Design review of the part built by this model. Coordinates are the model's own, in mm. A direction names the side the tool comes from. Coordinates: 2 decimals unless noted, no trailing zeros. Write each loop counter-clockwise with the first axis right and the second up, starting at its lowest first coordinate (ties: lowest second). Pieces come first, ordered by that corner, then holes.
Q1. Take a section at B-B, the plane x = -99. Write out the cut boundary in (y, z), plus the area to 3 significant figures.
Q2. For faces 1 (the flat face through (-185, -4, 5.452)), 2 (the flat face through (192.4, 0.1, -17.3)), 3 (the flat face through (177.6, 0.1, -0.1)), list the 3-axis set-ups (+Z, -Z, +X, -X, +Y, -Y) from which the entire face can be reached by the end or side of a thin tool; tool diameter is ignored.
Q3. The part is to be moulded in two halves that separate along Z. For faces 4 (the flat face through (-3, -3, -30)), 5 (the flat face through (187, -2, 5)), 6 (the flat face through (-3, 0, 30)), 7 (the flat face through (-3, 7.5, 3)), say which applies: released by +Z, released by -Z, zero draft, split by the parting line, or undercut.
Q4. For L1, parallel to Z at x = 182, y = -1.25; L2, parallel to Z at x = 152.5, y = 4; L3, parallel to Y at x = -55.5, z = -26.5, list the stretches that pass through material, from the lowest coordinate up.
Q5. For pin 1 Ø1 at (y, z) = (-4, -20) entering from +X; pin 2 Ø3 at (y, z) = (0.5, 20.5) entering from +X; pin 3 Ø1 at (y, z) = (0.5, 17.5) entering from -X, all flat-tipped, find the tip position at first contact; note any pin that passes through.
Q6. Take a section at A-A, the plane y = -0.25. Write out the cut boundary in (x, z), plus the area to 3 significant figures.
Q7. Take a section at C-C, the plane z = 13.5. Write out the cut boundary in (x, y), plus the area to 4 significant figures.
from build123d import *

# Parameters (mm, degrees)
F0_W     = 400
F0_H     = 60
F1_DEPTH = 7.5
F3_DEPTH = 60
F4_W     = 21.213203
F4_H     = 10
F5_DEPTH = 25
F6_W     = 21.213203
F6_H     = 10.904174
F7_DEPTH = 25
F8_W     = 5
F8_H     = 5
F9_DEPTH = 200


with BuildPart() as f1:
    # F0 (on Front) → F1 (new body, symmetric)
    with BuildSketch(Plane.XZ):
        Rectangle(F0_W, F0_H)
    extrude(amount=F1_DEPTH, both=True)

    # F2 (on face) → F3 (cut)
    with BuildSketch(Plane.XY.offset(30)):
        Polygon((-200, 7.5), (-200, -7.5), (-185, 7.5), align=None)
        Polygon((185, 7.5), (200, -7.5), (200, 7.5), align=None)
    extrude(amount=-F3_DEPTH, mode=Mode.SUBTRACT)

    # F4 (on face) → F5 (cut)
    with BuildSketch(Plane(origin=(96.25, 96.25, 0), x_dir=(-0.707107, 0.707107, 0), z_dir=(0.707107, 0.707107, 0))):
        with Locations((-136.118055, 0)):
            Rectangle(F4_W, F4_H)
    extrude(amount=-F5_DEPTH, mode=Mode.SUBTRACT)

    # F6 (on face) → F7 (cut)
    with BuildSketch(Plane(origin=(-96.25, 96.25, 0), x_dir=(-0.707107, -0.707107, 0), z_dir=(-0.707107, 0.707107, 0))):
        with Locations((136.118055, 0)):
            Rectangle(F6_W, F6_H)
    extrude(amount=-F7_DEPTH, mode=Mode.SUBTRACT)

    # F8 (on Right) → F9 (cut, symmetric)
    with BuildSketch(Plane.YZ):
        with Locations((5, -27.5)):
            Rectangle(F8_W, F8_H)
    extrude(amount=F9_DEPTH, both=True, mode=Mode.SUBTRACT)


solid = f1.part
Responses:
1. outline: (-7.5, -30) - (2.5, -30) - (2.5, -25) - (7.5, -25) - (7.5, 30) - (-7.5, 30) - close
1. area: 875 mm2
2. face 1: -X, -Y
2. face 2: +Z, -Z, +X, +Y
2. face 3: +X, -Y
3. face 4: released by -Z
3. face 5: undercut
3. face 6: released by +Z
3. face 7: zero draft
4. L1: z = -30 to -5, 5 to 30
4. L2: z = -25 to 30
4. L3: y = -7.5 to 2.5
5. pin 1: stops at x = 197
5. pin 2: stops at x = 193.5
5. pin 3: stops at x = -192.5
6. outline: (-192.75, -30) - (192.75, -30) - (192.75, -5) - (177.25, -5) - (177.25, 5) - (192.75, 5) - (192.75, 30) - (-192.75, 30) - (-192.75, 5.45) - (-177.25, 5.45) - (-177.25, -5.45) - (-192.75, -5.45) - close
6. area: 22,800 mm2
7. outline: (-200, -7.5) - (200, -7.5) - (185, 7.5) - (-185, 7.5) - close
7. area: 5,775 mm2
